from build123d import *

# Parameters (mm, degrees)
SKETCH_1_W          = 28
SKETCH_1_H          = 60
SKETCH_1_W_2        = 12
SKETCH_1_H_2        = 30
EXTRUDE_1_DEPTH     = 3
SKETCH_3_W          = 4
SKETCH_3_H          = 8
EXTRUDE_2_DEPTH     = 14
SKETCH_2_R          = 2
CUT_EXTRUDE_1_DEPTH = 12


with BuildPart() as part:
    # 草图1 → 凸台-拉伸1 (new, symmetric)
    with BuildSketch(Plane.XY):
        Rectangle(SKETCH_1_W, SKETCH_1_H)
        Rectangle(SKETCH_1_W_2, SKETCH_1_H_2, mode=Mode.SUBTRACT)
    extrude(amount=EXTRUDE_1_DEPTH, both=True)

    # 草图3 → 凸台-拉伸2 (add, symmetric)
    with BuildSketch(Plane(origin=(0, 0, 0), x_dir=(0, 0, -1), z_dir=(1, 0, 0))):
        with Locations((5, -26)):
            Rectangle(SKETCH_3_W, SKETCH_3_H)
        with Locations((5, 26)):
            Rectangle(SKETCH_3_W, SKETCH_3_H)
    extrude(amount=EXTRUDE_2_DEPTH, both=True)

    # 草图2 → 切除-拉伸1 (cut)
    with BuildSketch(Plane(origin=(0, 30, 0), x_dir=(1, 0, 0), z_dir=(0, 1, 0))):
        with Locations(Location((-9, 2, 0), (0, 0, 270))):
            Circle(SKETCH_2_R)
        with Locations(Location((9, 2, 0), (0, 0, 270))):
            Circle(SKETCH_2_R)
    cut_extrude_1 = extrude(amount=-CUT_EXTRUDE_1_DEPTH, mode=Mode.SUBTRACT)

    # 镜向1: 切除-拉伸1 across plane
    add(cut_extrude_1.mirror(Plane.ZX), mode=Mode.SUBTRACT)


solid = part.part
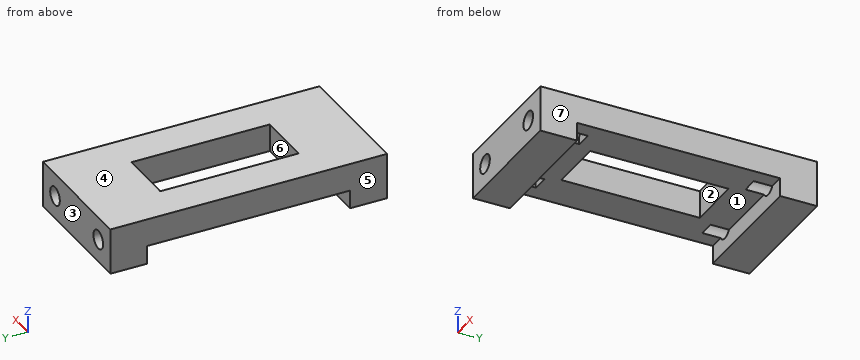
Here's how the part is built. I have some questions about the finished solid (model axes, mm). Face numbers are marked on the shaded views. A direction names the side the tool comes from. Coordinates: 2 decimals unless noted, no trailing zeros. Write each loop counter-clockwise with the first axis right and the second up, starting at its lowest first coordinate (ties: lowest second). Pieces come first, ordered by that corner, then holes.
1) I'm going to push flat-ended pins straight in: pin 1 (0.9 mm diameter, centred on x = -9, z = -1.5, fed in from +Y); pin 2 (1.5 mm diameter, centred on x = -8.5, z = -1, fed in from -Y); pin 3 (8 mm diameter, centred on x = -8.5, y = 15.5, fed in from -Z). Where does each tip first touch, or does it pass through?
Filled in:
pin 1: stops at y = 18
pin 2: stops at y = -18
pin 3: stops at z = -3
2) If we section it at D-D (x = 4): List the corners of the cut face in (y, z) for me, plus the area to 3 significant figures.
Filled in:
outline: (-30, -7) - (-22, -7) - (-22, -3) - (-15, -3) - (-15, 3) - (-30, 3) - close; (15, -3) - (22, -3) - (22, -7) - (30, -7) - (30, 3) - (15, 3) - close
area: 244 mm2
3) If we section it at C-C (z = 1.25): List the corners of the cut face in (x, y) for me.
Filled in:
outline: (-14, -30) - (14, -30) - (14, 30) - (-14, 30) - close; hole (-6, -15) - (6, -15) - (6, 15) - (-6, 15) - close
4) Thinking about a two-plate mould opening in X: for the marked faces 4, 5, 6 and 7, which applies, +X half, -X half, draft (parallel to the pull), parting line (faces both ways), or undercut?
Filled in:
face 4: draft
face 5: -X half
face 6: undercut
face 7: +X half
5) If we section it at B-B (x = 9): List the corners of the cut face in (y, z) for me.
Filled in:
outline: (-30, -7) - (-22, -7) - (-22, -4) - (-30, -4) - close; (-30, 0) - (-18, 0) - (-18, -3) - (18, -3) - (18, 0) - (30, 0) - (30, 3) - (-30, 3) - close; (22, -7) - (30, -7) - (30, -4) - (22, -4) - close
6) If we section it at A-A (z = -4.75): List the corners of the cut face in (x, y) for me, plus the area to 3 significant figures.
Filled in:
outline: (-14, -30) - (14, -30) - (14, -22) - (-14, -22) - close; (-14, 22) - (14, 22) - (14, 30) - (-14, 30) - close
area: 448 mm2
7) If I drill on line 1 (X direction, y = 24.5, z = -2); line 2 (Z direction, x = -9, y = -23); line 3 (Y direction, x = -5, z = -4), over which ranges is the centre line in solid material (lowest first)?
Filled in:
line 1: x = -14 to -11, -7 to 7, 11 to 14
line 2: z = -7 to -4, 0 to 3
line 3: y = -30 to -22, 22 to 30
8) Which directions (+Z, -Z, +X, -X, +Y, -Y) give clear straight access to the entire face, cutting with the end or side of a thin tool? Please do the marked faces 1, 2 and 3.
Filled in:
face 1: -Z, +X, -X
face 2: +Z, -Z
face 3: +Z, -Z, +X, -X, +Y
